Work out the finished part from the listing and answer in its coordinate system (mm). Face numbers are marked on the shaded views. A direction names the side the tool comes from. Coordinates: 2 decimals unless noted, no trailing zeros. Order: outer loops, then holes, each group sorted by start corner. A loop starts at its lowest first (then second) coordinate and runs counter-clockwise, first axis right, second up. Notation, with made-up numbers: M 24,14.25 L 32,14.25 A21 ccw 32,34.25 Z; hole C 67.5,6.25 d8. An arc over 180 degrees is marked long. Answer in a Markdown table with one row per item. Add a question column.
Item 1: The part is cut by section A-A (z = -33). Write down the section's boundary in (x, y), then the cut area to 3 significant figures.
Item 2: The part is cut by section D-D (z = 63.5). Write down the section's boundary in (x, y), then the cut area to 3 significant figures.
Item 3: Flat-ended cylindrical pins translate along their axes: pin 1 Ø8 at (y, z) = (193, 55.5) entering from -X; pin 2 Ø8 at (x, y) = (155.5, 194.5) entering from -Z. Find the tip coordinate at first contact, or state that the pin passes through.
Item 4: Consider line 1 (X direction, y = 208.5, z = 34.5); line 2 (Z direction, x = 128, y = 274.5); line 3 (Z direction, x = 177.5, y = 145.5). Determine where each line is inside the solid, lowest interval first. Write a range as from..to.
Item 5: Which of the six approach directions +Z, -Z, +X, -X, +Y, -Y give full straight-line access (tool end or side, diameter ignored) to the marked faces 4 and 5?
Item 6: The part is cut by section B-B (y = 67). Write down the section's boundary in (x, z).
Item 7: The mould has two halves that part along X. Classify the marked faces 1, 2 and 3: released by +X, released by -X, zero draft, split by the parting line, or undercut.
Item 8: The part is cut by section C-C (x = 152). Write down the section's boundary in (y, z).
from build123d import *

# Parameters (mm, degrees)
SKETCH4_W          = 722.984552569
SKETCH4_H          = 1077.767689397
CUT_EXTRUDE1_DEPTH = 3


with BuildPart() as part:
    # Sweep-Thin1: sweep along a path in Sketch3
    with BuildLine(Plane(origin=(0, 0, 0), x_dir=(0, 0, -1), z_dir=(1, 0, 0))) as sweep_thin1_path:
        Line((0, 0), (0, 300))
    # Sketch1 → Sweep-Thin1 (sweep)
    with BuildSketch(Plane(origin=(0, 0, 0), x_dir=(1, 0, 0), z_dir=(0, 1, 0))):
        with BuildLine():
            Line((-170, -78), (170, -78))
            ThreePointArc((170, -78), (193.334523779, -68.334523779), (203, -45))
            Line((203, -45), (203, 78))
            Line((203, 78), (-203, 78))
            Line((-203, 78), (-203, -45))
            ThreePointArc((-203, -45), (-193.334523779, -68.334523779), (-170, -78))
        make_face()
        with BuildLine():
            Line((-170, -75), (170, -75))
            ThreePointArc((170, -75), (191.213203436, -66.213203436), (200, -45))
            Line((200, -45), (200, 75))
            Line((200, 75), (-200, 75))
            Line((-200, 75), (-200, -45))
            ThreePointArc((-200, -45), (-191.213203436, -66.213203436), (-170, -75))
        make_face(mode=Mode.SUBTRACT)
    sweep(path=sweep_thin1_path.line)

    # Sketch4 → Cut-Extrude1 (cut)
    with BuildSketch(Plane(origin=(0, 0, -78), x_dir=(-1, 0, 0), z_dir=(0, 0, -1))):
        with Locations((86.276452511, -157.075497452)):
            Rectangle(SKETCH4_W, SKETCH4_H)
    extrude(amount=-CUT_EXTRUDE1_DEPTH, mode=Mode.SUBTRACT)


solid = part.part
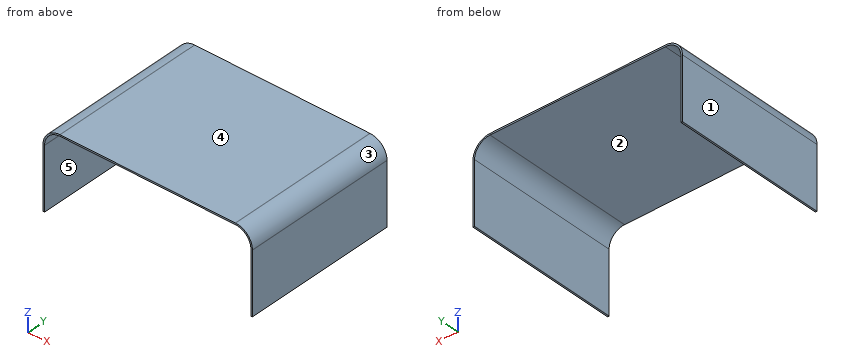
Reply:
| question | item | result |
|---|---|---|
| 1 | outline | M -203,0 L -200,0 L -200,300 L -203,300 Z; M 200,0 L 203,0 L 203,300 L 200,300 Z |
| 1 | area | 1,800 mm2 |
| 2 | outline | M -197.33,0 L -193.62,0 L -193.62,300 L -197.33,300 Z; M 193.62,0 L 197.33,0 L 197.33,300 L 193.62,300 Z |
| 2 | area | 2,230 mm2 |
| 3 | pin 1 | stops at x = -202.35 |
| 3 | pin 2 | stops at z = 75 |
| 4 | line 1 | x = -203..-200, 200..203 |
| 4 | line 2 | z = 75..78 |
| 4 | line 3 | z = 74.05..77.14 |
| 5 | face 4 | +Z, +X, -X, +Y, -Y |
| 5 | face 5 | -Z, +Y, -Y |
| 6 | outline | M -203,-75 L -200,-75 L -200,45 A30 cw -170,75 L 170,75 A30 cw 200,45 L 200,-75 L 203,-75 L 203,45 A33 ccw 170,78 L -170,78 A33 ccw -203,45 Z |
| 7 | face 1 | released by -X |
| 7 | face 2 | undercut |
| 7 | face 3 | released by +X |
| 8 | outline | M 0,75 L 300,75 L 300,78 L 0,78 Z |
